```python
from build123d import *

# Parameters (mm, degrees)
EXTRUDE_1_DEPTH             = 8
HOLE_WIZARD_M4_1_AT_2_COUNT = 2
HOLE_WIZARD_M4_1_AT_2_PITCH = 17.5
EXTRUDE_START               = -4
EXTRUDE_3_DEPTH             = 4
SKETCH_7_R                  = 4.5
CUT_EXTRUDE_1_DEPTH         = 1
SKETCH_8_R                  = 3.5
CUT_EXTRUDE_2_DEPTH         = 10
SKETCH_10_R                 = 4.5
CUT_EXTRUDE_3_DEPTH         = 17.170961718


with BuildPart() as part:
    # 草图1 → 凸台-拉伸1 (new body)
    with BuildSketch(Plane.XY):
        with BuildLine():
            Line((5.5, 0), (12.5, 0))
            Line((12.5, 0), (12.5, 3))
            Line((12.5, 3), (6.873863542, 3))
            ThreePointArc((6.873863542, 3), (0, 7.5), (-6.873863542, 3))
            Line((-6.873863542, 3), (-12.5, 3))
            Line((-12.5, 3), (-12.5, 0))
            Line((-12.5, 0), (-5.5, 0))
            Line((-5.5, 0), (-5.5, -0.5))
            Line((-5.5, -0.5), (-4.00894001, -0.5))
            ThreePointArc((-4.00894001, -0.5), (0, 4.04), (4.00894001, -0.5))
            Line((4.00894001, -0.5), (5.5, -0.5))
            Line((5.5, -0.5), (5.5, 0))
        make_face()
    extrude(amount=EXTRUDE_1_DEPTH)

    # 草图5 → M4 间隙孔1 (revolve, cut)
    with BuildSketch(Plane(origin=(-8.75, 3, 4), x_dir=(0, 0, 1), z_dir=(1, 0, 0))):
        Polygon((0, 0), (0, 4.501936393), (2.25, 3.15), (2.25, 0.025), (2.275, 0), align=None)
    hole_wizard_m4_1 = revolve(axis=Axis((-8.75, 9.35, 4), (0, -1, 0)), mode=Mode.SUBTRACT)

    # M4 间隙孔1 at 2: M4 间隙孔1 ×2
    with Locations(*[(i * HOLE_WIZARD_M4_1_AT_2_PITCH, 0, 0) for i in range(1, HOLE_WIZARD_M4_1_AT_2_COUNT)]):
        add(hole_wizard_m4_1, mode=Mode.SUBTRACT)

    # 草图6 → 凸台-拉伸3 (add)
    with BuildSketch(Plane.XY.offset(8).offset(EXTRUDE_START)):
        with BuildLine():
            Line((-4.00894001, -0.5), (-3.464101615, -0.5))
            ThreePointArc((-3.464101615, -0.5), (0, 3.5), (3.464101615, -0.5))
            Line((3.464101615, -0.5), (4.00894001, -0.5))
            ThreePointArc((4.00894001, -0.5), (0, 4.04), (-4.00894001, -0.5))
        make_face()
    extrude(amount=EXTRUDE_3_DEPTH)

    # 草图7 → 切除-拉伸1 (cut)
    with BuildSketch(Plane(origin=(0, 0, 0), x_dir=(-1, 0, 0), z_dir=(0, 0, -1))):
        Circle(SKETCH_7_R)
    extrude(amount=-CUT_EXTRUDE_1_DEPTH, mode=Mode.SUBTRACT)

    # 草图8 → 切除-拉伸2 (cut)
    with BuildSketch(Plane(origin=(0, 3, 0), x_dir=(1, 0, 0), z_dir=(0, 1, 0))):
        with Locations((-8.75, -4)):
            Circle(SKETCH_8_R)
    cut_extrude_2 = extrude(amount=CUT_EXTRUDE_2_DEPTH, mode=Mode.SUBTRACT)

    # 镜向1: 切除-拉伸2 across plane
    add(cut_extrude_2.mirror(Plane(origin=(0, 0, 0), x_dir=(0, 0, 1), z_dir=(1, 0, 0))), mode=Mode.SUBTRACT)

    # 草图10 → 切除-拉伸3 (cut, through all)
    with BuildSketch(Plane(origin=(0, 0, 1), x_dir=(-1, 0, 0), z_dir=(0, 0, -1))):
        Circle(SKETCH_10_R)
    extrude(amount=-CUT_EXTRUDE_3_DEPTH, mode=Mode.SUBTRACT)


solid = part.part
```
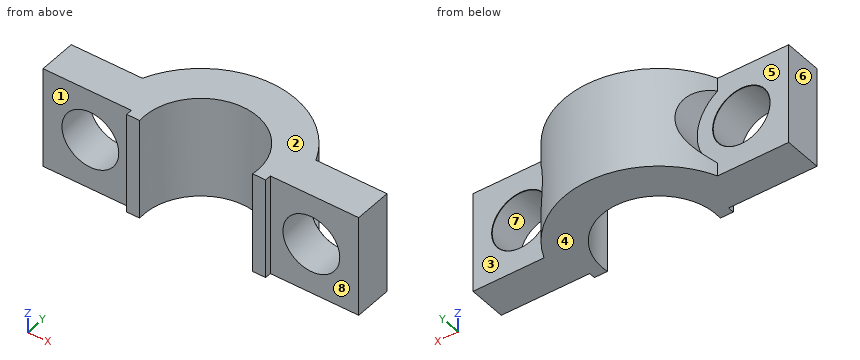
Input: part model. Units: mm. Frame: model coordinates. Face numbers are marked on the shaded views. A direction names the side the tool comes from. Round coordinates to 2 decimals unless told otherwise and drop trailing zeros. Loops run counter-clockwise (first coordinate to the right, second up) from the corner with the lowest first, then second, coordinate; pieces in that order, holes last. Notation, with made-up numbers: (21.5, -28) - (62.5, -28) arc R25 cw to (62.5, -7) - close; hole circle Ø6 at (48.5, -18.75). An arc over 180 degrees is marked (long way). One line per item, written item: value. Start each with the question number.
(1) Section B-B, the plane y = 1.5. Return loops of the section in (x, z).
(2) Contact query for flat-ended pins moving along their axis: P1, Ø3, axis at x = 9.5, z = 7, coming from the -Y side; P2, Ø2, axis at x = -7.5, z = 5, coming from the +Y side. Output: stop coordinate, or through.
(3) Draft query along X for the marked faces 6, 7 and 8. Return one class per face: +X half, -X half, draft (parallel to the pull), parting line (faces both ways), or undercut.
(4) Access query for the marked faces 1, 2, 3, 4 and 5. Directions: +Z, -Z, +X, -X, +Y, -Y. A direction counts if a zero-diameter tool reaches every point of the face in a straight line with its end or side. Return the directions, or none.
(5) Section D-D, the plane x = 0. Return loops of the section in (y, z), plus the area to 3 significant figures.
(6) Section A-A, the plane x = 8.75. Return loops of the section in (y, z) (3 decimals).
(7) Ray query, line 1 (Z direction, x = 8.75, y = 2.2); line 2 (X direction, y = 1.1, z = 4); line 3 (X direction, y = 0.5, z = 3.75). Return the intervals inside material, ascending. Write a range as [from, to].
(8) Section C-C, the plane z = 4. Return loops of the section in (x, y) (3 decimals).
Results below:
1. outline: (-12.5, 0) - (-4.24, 0) - (-4.24, 8) - (-12.5, 8) - close; (4.24, 0) - (12.5, 0) - (12.5, 8) - (4.24, 8) - close; hole circle Ø4.5 at (-8.75, 4); hole circle Ø4.5 at (8.75, 4)
2. P1: y = 0
2. P2: y = 3
3. face 6: -X half
3. face 7: undercut
3. face 8: draft
4. face 1: +Z, -Z, -X, -Y
4. face 2: +Z, +X, -X, +Y, -Y
4. face 3: +X, +Y
4. face 4: -Z, +X, -X, +Y, -Y
4. face 5: -X, +Y
5. outline: (4.5, 0) - (7.5, 0) - (7.5, 8) - (4.5, 8) - close
5. area: 24.0 mm^2
6. outline: (0, 0) - (3, 0) - (3, 1.725) - (2.975, 1.75) - (0, 1.75) - close; (0, 6.25) - (2.975, 6.25) - (3, 6.275) - (3, 8) - (0, 8) - close
7. line 1: [0, 1.75], [6.25, 8]
7. line 2: [-12.5, -11], [-6.5, -4.36], [4.36, 6.5], [11, 12.5]
7. line 3: [-12.5, -10.99], [-6.51, -4.47], [4.47, 6.51], [10.99, 12.5]
8. outline: (-12.5, 0) - (-11, 0) - (-11, 2.975) - (-11.025, 3) - (-12.5, 3) - close; (-6.5, 0) - (-5.5, 0) - (-5.5, -0.5) - (-4.472, -0.5) arc R4.5 cw (long way) to (4.472, -0.5) - (5.5, -0.5) - (5.5, 0) - (6.5, 0) - (6.5, 2.975) - (6.475, 3) - (5.25, 3) - (5.25, 5.356) arc R7.5 ccw to (-5.25, 5.356) - (-5.25, 3) - (-6.475, 3) - (-6.5, 2.975) - close; (11, 0) - (12.5, 0) - (12.5, 3) - (11.025, 3) - (11, 2.975) - close
